Work out the finished part from the listing and answer in its coordinate system (mm). Coordinates: 2 decimals unless noted, no trailing zeros. Order: outer loops, then holes, each group sorted by start corner. A loop starts at its lowest first (then second) coordinate and runs counter-clockwise, first axis right, second up.
1. Determine the mould class of faces 1 (the cylindrical face through (-1.86, 36.518, 2.576)), 2 (the cylindrical face through (55.34, 99.69, 2.58)), 3 (the flat face through (-1, 1, 5.08)), 4 (the cylindrical face through (-25.47, -94.68, 2.58)) for opening direction X: +X half, -X half, draft (parallel to the pull), parting line (faces both ways), or undercut.
2. A flat-ended cylindrical pin translates along its axis: pin 1 Ø17 at (x, y) = (0, 22.352) entering from -Z. Find the tip coordinate at first contact, or state that the pin passes through.
3. Find the intervals of material crossed by probe 1 along X at (y, z) = (-91, 4.55); probe 2 along Y at (x, z) = (10.16, 3); probe 3 along Y at (x, z) = (0, 3.15), in increasing order.
4. The part is cut by section A-A, the plane x = 0. Give the vertices of the cut face in (y, z).
5. The part is cut by section B-B, the plane z = 2. Count the separate pieces of the cut face and the enclosed holes in it, then the cut area to 3 significant figures.
```python
from build123d import *

# Parameters (mm, degrees)
SKETCH1_W           = 114.3
SKETCH1_H           = 203.2
BOSS_EXTRUDE1_DEPTH = 5.08
FILLET1_R           = 6.35
SKETCH3_R           = 14.2875
CUT_EXTRUDE1_DEPTH  = 5.08
SKETCH4_R           = 2.667
CUT_EXTRUDE2_DEPTH  = 5.08


with BuildPart() as part:
    # Sketch1 → Boss-Extrude1 (new body)
    with BuildSketch(Plane.XY):
        Rectangle(SKETCH1_W, SKETCH1_H)
    extrude(amount=BOSS_EXTRUDE1_DEPTH)

    # Fillet1
    fillet1_edges = [part.edges().sort_by_distance(p)[0] for p in [
        (-57.15, 101.6, 2.54),
        (57.15, 101.6, 2.54),
    ]]
    fillet(fillet1_edges, radius=FILLET1_R)

    # Sketch3 → Cut-Extrude1 (cut)
    with BuildSketch(Plane.XY.offset(5.08)):
        with Locations((0, 22.352)):
            Circle(SKETCH3_R)
    extrude(amount=-CUT_EXTRUDE1_DEPTH, mode=Mode.SUBTRACT)

    # Sketch4 → Cut-Extrude2 (cut)
    with BuildSketch(Plane.XY.offset(5.08)):
        with Locations((10.16, -92.075)):
            Circle(SKETCH4_R)
        with Locations((-24.892, -92.075)):
            Circle(SKETCH4_R)
    extrude(amount=-CUT_EXTRUDE2_DEPTH, mode=Mode.SUBTRACT)


solid = part.part
```
Geometry says:
1. face 1: undercut
1. face 2: +X half
1. face 3: draft
1. face 4: undercut
2. pin 1: passes through
3. probe 1: x = -57.15 to -27.33, -22.45 to 7.72, 12.6 to 57.15
3. probe 2: y = -101.6 to -94.74, -89.41 to 12.31, 32.4 to 101.6
3. probe 3: y = -101.6 to 8.06, 36.64 to 101.6
4. outline: (-101.6, 0) - (8.06, 0) - (8.06, 5.08) - (-101.6, 5.08) - close; (36.64, 0) - (101.6, 0) - (101.6, 5.08) - (36.64, 5.08) - close
5. separate pieces: 1
5. enclosed holes: 3
5. area: 22,500 mm2
